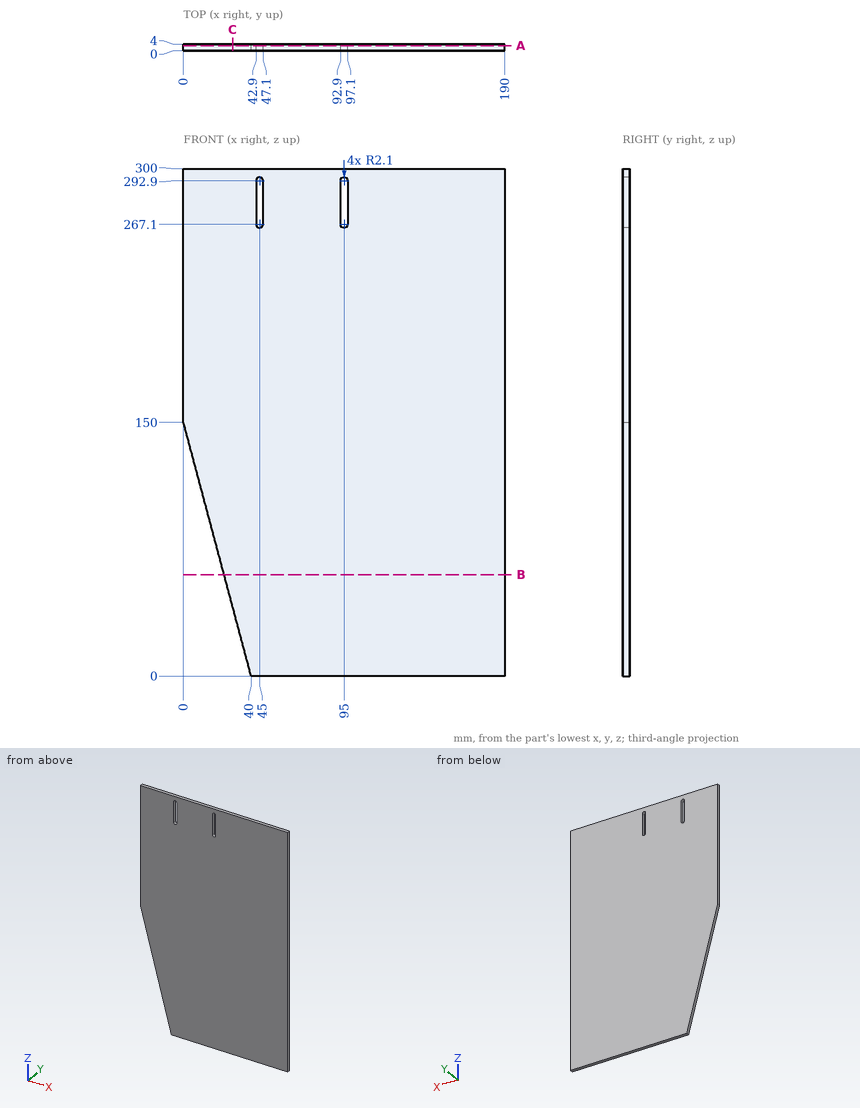
Study the drawing (mm; zero at the part's minimum x, y, z) and answer. Coordinates: 2 decimals unless noted, no trailing zeros. Write each loop counter-clockwise with the first axis right and the second up, starting at its lowest first coordinate (ties: lowest second). Pieces come first, ordered by that corner, then holes. Notation, with made-up numbers: (47.5, -31) - (88.5, -31) arc R11 cw to (88.5, -12) - close; hole circle Ø7 at (-4, -13). An arc over 180 degrees is marked (long way). One line per item, written item: value.
1) Consider line 1 along X through (y, z) = (1.4, 278); line 2 along X through (y, z) = (1.95, 39); line 3 along X through (y, z) = (3.3, 78.5). Determine where each line is inside the solid, lowest interval first. Write a range as from..to.
Geometry check:
line 1: x = 0..42.9, 47.1..92.9, 97.1..190
line 2: x = 29.6..190
line 3: x = 19.07..190
2) Find section B-B (z = 60). Give the vertices of the cut face in (x, y).
Geometry check:
outline: (24, 0) - (190, 0) - (190, 4) - (24, 4) - close
3) Find section C-C (x = 29). Give the vertices of the cut face in (y, z), and give its area (4 significant figures).
Geometry check:
outline: (0, 41.25) - (4, 41.25) - (4, 300) - (0, 300) - close
area: 1,035 mm2
4) Find section A-A (y = 3.1). Give the vertices of the cut face in (x, z), and give its area (3 significant figures).
Geometry check:
outline: (0, 150) - (40, 0) - (190, 0) - (190, 300) - (0, 300) - close; hole (42.9, 267.1) arc R2.1 ccw to (47.1, 267.1) - (47.1, 292.9) arc R2.1 ccw to (42.9, 292.9) - close; hole (92.9, 267.1) arc R2.1 ccw to (97.1, 267.1) - (97.1, 292.9) arc R2.1 ccw to (92.9, 292.9) - close
area: 53,800 mm2
